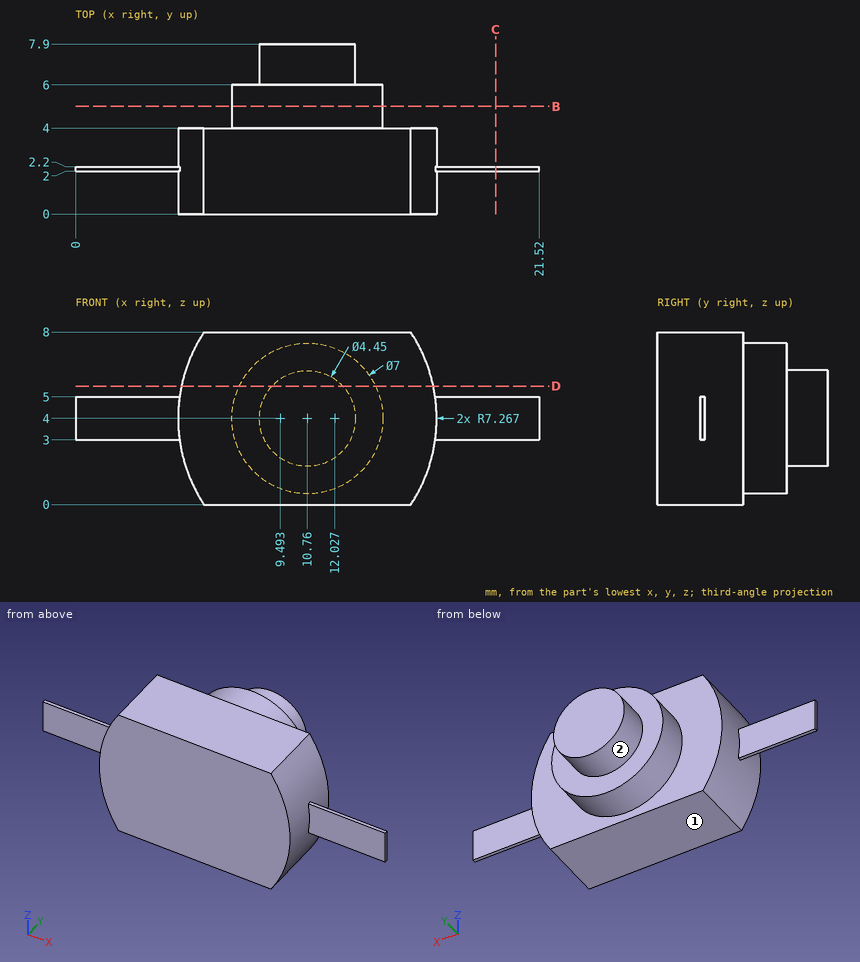
Could you check a few things on this drawing? It's one solid part, dimensions in mm from its lowest x, y, z. A direction names the side the tool comes from. Give positions to 0.01 mm unless a question says otherwise; leave off trailing zeros. Order: outer loops, then holes, each group sorted by start corner. A loop starts at its lowest first (then second) coordinate and runs counter-clockwise, first axis right, second up. Notation, with made-up numbers: (45.5, 22.5) -> (92.5, 22.5) arc R21 ccw to (92.5, 29.5) -> close; hole circle Ø5 at (-21, -26). An arc over 180 degrees is marked (long way). Answer in a Markdown table with one row per item. Add a question column.
Item 1: Imagine slicing it at C-C (x = 19.5). List the corners of the cut face in (y, z) for me.
Item 2: For the marked faces 1 and 2, which set-ups out of +Z, -Z, +X, -X, +Y, -Y let a thin tool reach every point of the face, with its end or its side?
Item 3: Imagine slicing it at D-D (z = 5.5). List the corners of the cut face in (x, y) for me.
Item 4: Imagine slicing it at B-B (y = 5). List the corners of the cut face in (x, z) for me.
Item 5: Please list where these lines run through material, in increasing order: probe 1 along Y at (x, z) = (1.5, 4); probe 2 along X at (y, z) = (1.25, 4); probe 3 along Y at (x, z) = (16, 1.25).
Item 6: I'm going to push flat-ended pins straight in: P1, Ø4, axis at x = 7, z = 7, coming from the +Y side; P2, Ø1.5, axis at y = 6, z = 5, coming from the -X side; P3, Ø0.6, axis at x = 2.5, z = 4, coming from the +Y side. Where does each tip first touch, or does it pass through?
Result:
| question | item | result |
|---|---|---|
| 1 | outline | (2, 3) -> (2.2, 3) -> (2.2, 5) -> (2, 5) -> close |
| 2 | face 1 | -Z, +X, -X, +Y, -Y |
| 2 | face 2 | +Y |
| 3 | outline | (4.92, 0) -> (16.6, 0) -> (16.6, 4) -> (13.92, 4) -> (13.92, 6) -> (12.4, 6) -> (12.4, 7.9) -> (9.12, 7.9) -> (9.12, 6) -> (7.6, 6) -> (7.6, 4) -> (4.92, 4) -> close |
| 4 | outline | circle Ø7 at (10.76, 4) |
| 5 | probe 1 | 2 to 2.2 |
| 5 | probe 2 | 4.76 to 16.76 |
| 5 | probe 3 | 0 to 4 |
| 6 | P1 | y = 6 |
| 6 | P2 | x = 7.27 |
| 6 | P3 | y = 2.2 |
